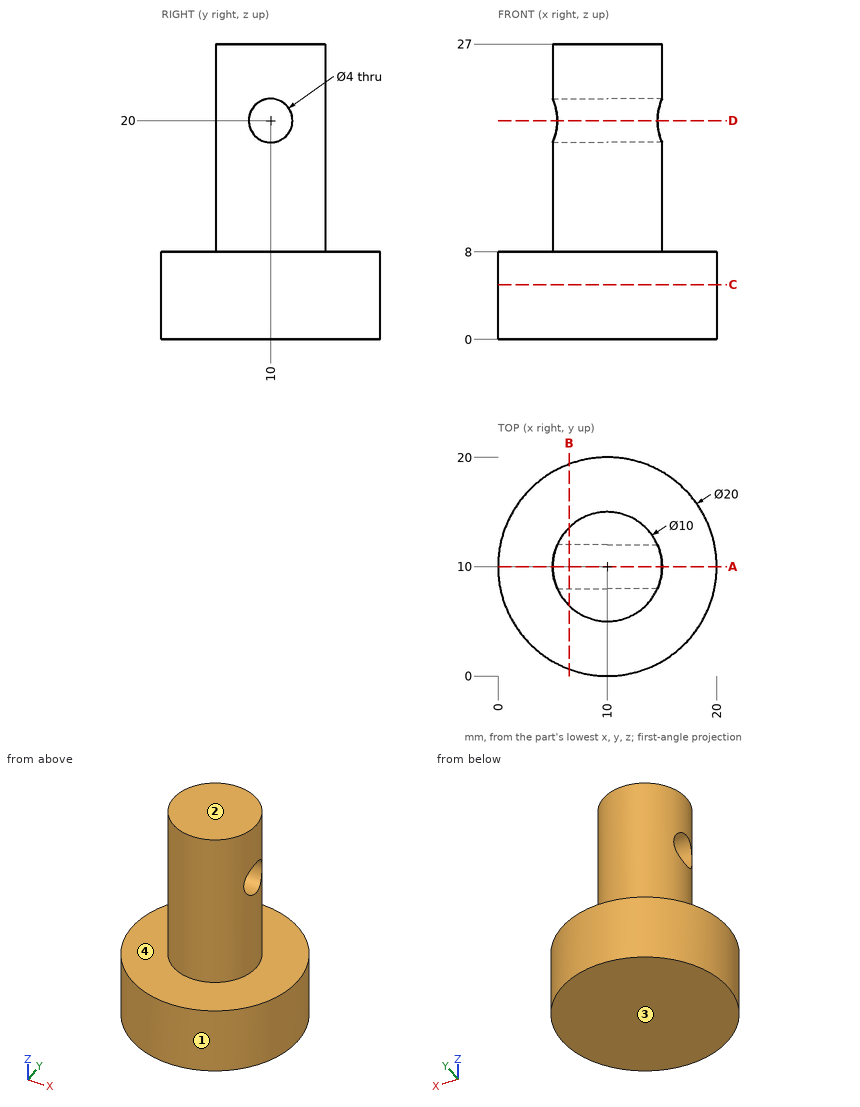
Verification items for this drawing (mm, ordinates from the low corner). A direction names the side the tool comes from. Round coordinates to 2 decimals unless told otherwise and drop trailing zeros. Order: outer loops, then holes, each group sorted by start corner. A loop starts at its lowest first (then second) coordinate and runs counter-clockwise, first axis right, second up. Notation, with made-up numbers: M -19,-37.5 L 22,-37.5 A32 ccw 22,0.5 Z; hole C 43.25,-1 d2. An arc over 180 degrees is marked long. Answer in a Markdown table with one row per item. Add a question column.
Item 1: Sectioned sample at D-D, the plane z = 20. Enter the section's corners in (x, y).
Item 2: Draft check along X on the marked faces 1 and 2. Enter one of: released by +X, released by -X, zero draft, split by the parting line, or undercut.
Item 3: Sectioned sample at C-C, the plane z = 5. Enter the section's corners in (x, y).
Item 4: Material ranges on L1, parallel to Z at x = 12.85, y = 10; L2, parallel to Z at x = 7, y = 14.25; L3, parallel to X at y = 9.75, z = 10.5, recorded low to high. Write a range as [from, to].
Item 5: Depth check by flat-ended pin: pin 1 Ø12 at (y, z) = (9.5, 10) entering from +X; pin 2 Ø4 at (x, z) = (15, 23) entering from -Y; pin 3 Ø10 at (y, z) = (17.5, 14) entering from +X; pin 4 Ø12 at (x, z) = (8, 20) entering from +Y. Enter the tip coordinate at first touch or a pass-through.
Item 6: Set-up check for the marked faces 3 and 4: record each of +Z, -Z, +X, -X, +Y, -Y from which the full face is reachable in a straight line by a thin tool's end or side.
Item 7: Sectioned sample at A-A, the plane y = 10. Enter the section's corners in (x, z).
Item 8: Sectioned sample at B-B, the plane x = 6.5. Enter the section's corners in (y, z).
Filled in:
| question | item | result |
|---|---|---|
| 1 | outline | M 5.42,8 A5 ccw 14.58,8 Z; M 5.42,12 L 14.58,12 A5 ccw Z |
| 2 | face 1 | split by the parting line |
| 2 | face 2 | zero draft |
| 3 | outline | C 10,10 d20 |
| 4 | L1 | z = [0, 18], [22, 27] |
| 4 | L2 | z = [0, 8] |
| 4 | L3 | x = [5.01, 14.99] |
| 5 | pin 1 | stops at x = 20 |
| 5 | pin 2 | stops at y = 6 |
| 5 | pin 3 | stops at x = 14.33 |
| 5 | pin 4 | stops at y = 15 |
| 6 | face 3 | -Z, +X, -X, +Y, -Y |
| 6 | face 4 | +Z |
| 7 | outline | M 0,0 L 20,0 L 20,8 L 15,8 L 15,18 L 5,18 L 5,8 L 0,8 Z; M 5,22 L 15,22 L 15,27 L 5,27 Z |
| 8 | outline | M 0.63,0 L 19.37,0 L 19.37,8 L 13.57,8 L 13.57,27 L 6.43,27 L 6.43,8 L 0.63,8 Z; hole C 10,20 d4 |
